from build123d import *

# Parameters (mm, degrees)
F2_R     = 6.782292
F3_DEPTH = 10.16
F4_R     = 4.804255
F5_DEPTH = 4


with BuildPart() as f1:
    # F0 (on Front) → F1 (revolve)
    with BuildSketch(Plane.XZ):
        with BuildLine():
            Line((0, 41.822274), (0, -21.52941))
            Line((0, -21.52941), (16.948683, -21.52941))
            Line((16.948683, -21.52941), (16.948683, 44.362274))
            Line((16.948683, 44.362274), (2.54, 44.362274))
            ThreePointArc((2.54, 44.362274), (0.743949, 43.618325), (0, 41.822274))
        make_face()
    revolve(axis=Axis((16.948683, 0, 11.416432), (0, 0, 1)))

    # F2 (on face) → F3 (join)
    with BuildSketch(Plane.XY.offset(44.362274)):
        with Locations((16.948683, 0)):
            Circle(F2_R)
    extrude(amount=F3_DEPTH)

    # F4 (on face) → F5 (join)
    with BuildSketch(Plane.XY.offset(54.522274)):
        with Locations((16.948683, 0)):
            Circle(F4_R)
    extrude(amount=-F5_DEPTH)


solid = f1.part
Check sheet for the modelled part. Datum: model origin and axes. Units: mm. A direction names the side the tool comes from. Round coordinates to 2 decimals unless told otherwise and drop trailing zeros. Loops run counter-clockwise (first coordinate to the right, second up) from the corner with the lowest first, then second, coordinate; pieces in that order, holes last.
1. Scan lines: probe 1 along Y at (x, z) = (8, 41); probe 2 along Z at (x, y) = (16, 8.5); probe 3 along Y at (x, z) = (13.5, -14). Record each from-to range of solid material in increasing order.
2. Sectioned sample at B-B on z = 2.5. Record the boundary of the cut face in (x, y).
3. Gauge pin test, flat ends, axial feed: pin 1 Ø3 at (x, y) = (13, 12) entering from +Z; pin 2 Ø1.5 at (x, z) = (15, 36.5) entering from +Y. Record the tip position at first contact, or that the pin passes through.
4. Set-up check for faces 1 (the flat face through (17, 0, 54.522)), 2 (the cylindrical face through (23.418, 2.037, 49.371)): record each of +Z, -Z, +X, -X, +Y, -Y from which the full face is reachable in a straight line by a thin tool's end or side.
5. Sectioned sample at A-A on y = 0. Record the boundary of the cut face in (x, z), and give its area (3 significant figures).
Recorded:
1. probe 1: y = -14.39 to 14.39
1. probe 2: z = -21.53 to 44.36
1. probe 3: y = -16.59 to 16.59
2. outline: circle Ø33.9 at (16.95, 0)
3. pin 1: stops at z = 44.36
3. pin 2: stops at y = 16.91
4. face 1: +Z, +X, -X, +Y, -Y
4. face 2: +Z
5. outline: (0, -21.53) - (33.9, -21.53) - (33.9, 41.82) arc R2.54 ccw to (31.36, 44.36) - (23.73, 44.36) - (23.73, 54.52) - (10.17, 54.52) - (10.17, 44.36) - (2.54, 44.36) arc R2.54 ccw to (0, 41.82) - close
5. area: 2,370 mm2
